Input: part model. Units: mm. Frame: model coordinates. Face numbers are marked on the shaded views. Give positions to 0.01 mm unless a question says otherwise; leave off trailing zeros. Loops run counter-clockwise (first coordinate to the right, second up) from the corner with the lowest first, then second, coordinate; pieces in that order, holes last. Notation, with made-up numbers: M 30.25,-3 L 72.25,-3 A8 cw 72.25,4 Z; hole C -35,7.25 d11. An arc over 180 degrees is marked long. Use a Markdown table: item, result. Add a question column.
from build123d import *

# Parameters (mm, degrees)
SKETCH008_R     = 30
PAD004_DEPTH    = 5
SKETCH009_R     = 40
SKETCH009_R_2   = 35
POCKET002_DEPTH = 3
SKETCH015_R     = 1.75
POCKET008_DEPTH = 5
SKETCH038_W     = 13.2
SKETCH038_H     = 2.5
PAD009_DEPTH    = 1


with BuildPart() as part:
    # Sketch008 → Pad004 (new body)
    with BuildSketch(Plane.XY):
        Circle(SKETCH008_R)
    extrude(amount=PAD004_DEPTH)

    # Sketch009 (on Face3 of Pad004) → Pocket002 (cut)
    with BuildSketch(Plane.XY.offset(5)):
        with Locations((-50, 0)):
            Circle(SKETCH009_R)
        with Locations((-50, 0)):
            Circle(SKETCH009_R_2, mode=Mode.SUBTRACT)
    extrude(amount=-POCKET002_DEPTH, mode=Mode.SUBTRACT)

    # Sketch015 (on Face3 of Pocket002) → Pocket008 (cut)
    with BuildSketch(Plane.XY.offset(5)):
        with Locations((-24, 0)):
            Circle(SKETCH015_R)
        with Locations((14.520833, 19.108778)):
            Circle(SKETCH015_R)
        with Locations((14.520833, -19.108778)):
            Circle(SKETCH015_R)
    extrude(amount=-POCKET008_DEPTH, mode=Mode.SUBTRACT)

    # Sketch038 (on Face3 of Pocket008) → Pad009 (join)
    with BuildSketch(Plane.XY.offset(5)):
        with Locations((0, 17.25)):
            Rectangle(SKETCH038_W, SKETCH038_H)
    extrude(amount=PAD009_DEPTH)


solid = part.part
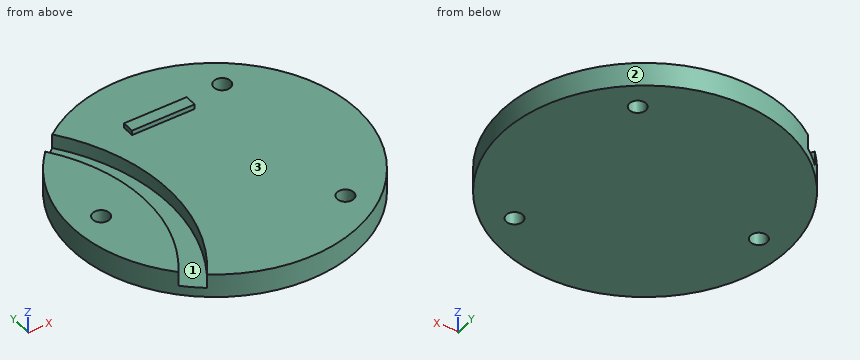
1) Pull-direction query (X, two-part tool) for the marked faces 1, 2 and 3; classes: pulls with the +X half, pulls with the -X half, needs draft (parallel to the pull), parting line crosses it, or undercut.
2) Section query C-C, the plane x = -24. Return the cut outline in (y, z).
3) Section query D-D, the plane x = 0. Return the cut outline in (y, z), and give its area (4 significant figures).
4) Section query B-B, the plane z = 3.8. Return the cut outline in (x, y).
5) Contact query for flat-ended pins moving along their axis: P1, Ø1.1, axis at x = -0.5, z = 5.5, coming from the -Y side; P2, Ø13, axis at x = -18.5, y = 9.5, coming from the +Z side; P3, Ø3, axis at x = 14.52, y = 19.11, coming from the -Z side; P4, Ø0.8, axis at y = 17.5, z = 5.5, coming from the -X side. Output: stop coordinate, or through.
6) Ray query, line 1 (X direction, y = -20, z = 4.15); line 2 (Z direction, x = -7, y = -5); line 3 (Y direction, x = 0.5, z = 1.5). Return the intervals inside material, ascending. Write a range as [from, to].
7) Section query A-A, the plane y = 0. Return the cut outline in (x, z), and give its area (4 significant figures).
Entries:
| question | item | result |
|---|---|---|
| 1 | face 1 | undercut |
| 1 | face 2 | parting line crosses it |
| 1 | face 3 | needs draft |
| 2 | outline | M -18,0 L -1.75,0 L -1.75,5 L -18,5 Z; M 1.75,0 L 18,0 L 18,5 L 1.75,5 Z |
| 3 | outline | M -30,0 L 30,0 L 30,5 L 18.5,5 L 18.5,6 L 16,6 L 16,5 L -30,5 Z |
| 3 | area | 302.5 mm² |
| 4 | outline | M -21.75,-20.66 A35 ccw -21.75,20.66 A30 ccw Z; M -18,-24 A30 ccw long -18,24 A40 cw Z; hole C -24,0 d3.5; hole C 14.52,-19.11 d3.5; hole C 14.52,19.11 d3.5 |
| 5 | P1 | stops at y = -30 |
| 5 | P2 | stops at z = 5 |
| 5 | P3 | passes through |
| 5 | P4 | stops at x = -6.6 |
| 6 | line 1 | x = [-22.36, -21.28], [-15.36, 13.01], [16.03, 22.36] |
| 6 | line 2 | z = [0, 5] |
| 6 | line 3 | y = [-30, 30] |
| 7 | outline | M -30,0 L -25.75,0 L -25.75,5 L -30,5 Z; M -22.25,0 L 30,0 L 30,5 L -10,5 L -10,2 L -15,2 L -15,5 L -22.25,5 Z |
| 7 | area | 267.5 mm² |
